For this review, take the finished solid that the model builds, in its own axes (mm). A direction names the side the tool comes from. Round coordinates to 2 decimals unless told otherwise and drop trailing zeros. Write each loop counter-clockwise with the first axis right and the second up, starting at its lowest first coordinate (ties: lowest second). Pieces come first, ordered by that corner, then holes. Notation, with made-up numbers: (-17.5, 67) -> (5.5, 67) arc R13 ccw to (5.5, 83) -> close; hole circle Ø10 at (49.25, 2.25). An arc over 180 degrees is marked (long way). Answer in a Markdown table with one row per item.
Autodesk Inventor part; units mm, degrees
ref_plane "YZ Plane" through (0, 0, 0) normal (1, 0, 0) x (0, 1, 0)
ref_plane "XZ Plane" through (0, 0, 0) normal (0, 1, 0) x (-1, 0, 0)
ref_plane "XY Plane" through (0, 0, 0) normal (0, 0, 1) x (1, 0, 0)
sketch "Sketch1" plane through (0, 0, 0) normal (0, 0, 1) x (1, 0, 0)
  line L0 (0, 0) -> (100, 0)
  line L1 (100, 0) -> (100, 39)
  line L2 (100, 39) -> (0, 39)
  line L3 (0, 39) -> (0, 0)
  dimension "d45" = 100
  dimension "d46" = 39
extrude "bottom" add sketch "Sketch1" along normal blind 3
sketch "Sketch5" plane through (0, 0, 0) normal (0, 0, -1) x (-1, 0, 0)
  line L0 (0, 0) -> (-100, 0)
  line L1 (0, 39) -> (0, 0)
  line L2 (-100, 39) -> (0, 39)
  line L3 (-100, 0) -> (-100, 39)
  line L4 (3, 42) -> (3, -3)
  line L5 (3, -3) -> (-103, -3)
  line L6 (-103, -3) -> (-103, 42)
  line L7 (-103, 42) -> (3, 42)
  dimension "d30" = 3
extrude "walls" add sketch "Sketch5" against normal blind 19.6
sketch "holes" plane through (0, 0, 0) normal (0, 0, 1) x (1, 0, 0)
  line L0 (0, 0) -> (100, 0)
  line L1 (100, 0) -> (100, 39)
  line L2 (100, 39) -> (0, 39)
  line L3 (0, 39) -> (0, 0)
  circle A0 centre (21.5, 34.5) radius 1.55 construction
  circle A1 centre (96.5, 34.5) radius 1.55 construction
  circle A2 centre (96.5, 3.5) radius 1.55 construction
  circle A3 centre (21.5, 3.5) radius 1.55 construction
  line L4 (21.5, 34.5) -> (21.5, 3.5) construction
  line L5 (21.5, 3.5) -> (96.5, 3.5) construction
  line L6 (96.5, 3.5) -> (96.5, 34.5) construction
  line L7 (96.5, 34.5) -> (21.5, 34.5) construction
  dimension "d33" = 3.1
  dimension "d34" = 75
  dimension "d35" = 31
  dimension "d50" = 3.5
  dimension "d51" = 3.5
sketch "Sketch8" plane through (0, 0, 0) normal (0, 0, -1) x (-1, 0, 0)
  line L0 (-95, 6.3) -> (-23, 6.3)
  line L1 (-23, 6.3) -> (-23, 31)
  line L2 (-23, 31) -> (-95, 31)
  line L3 (-95, 31) -> (-95, 6.3)
  line L4 (3, -3) -> (-103, -3)
  line L5 (-96.5, 3.5) -> (-96.5, 34.5) construction
  line L6 (-21.5, 34.5) -> (-21.5, 3.5) construction
  point P0 (0, 0)
  dimension "d99" = 1.5
  dimension "d100" = 1.5
  dimension "d101" = 3.5
  dimension "d102" = 2.8
extrude "display" cut sketch "Sketch8" along normal through all both and the other way through all
sketch "Sketch7" plane through (0, 0, 3) normal (0, 0, 1) x (1, 0, 0)
  circle A0 centre (96.5, 34.5) radius 1.55 construction
  circle A1 centre (21.5, 3.5) radius 1.55 construction
  circle A2 centre (21.5, 34.5) radius 1.55 construction
  arc A3 (23.4365, 31) -> (25.5, 34.5) centre (21.5, 34.5) ccw
  line L0 (15.5, 39) -> (27.5, 39)
  line L1 (0, 39) -> (100, 39)
  arc A4 (27.5, 39) -> (25.5, 37) centre (27.5, 37) ccw
  line L2 (25.5, 37) -> (25.5, 34.5)
  line L3 (16.3235, 0) -> (26.6765, 0)
  line L4 (23, 31) -> (95, 31) construction
  arc A5 (92.6921, 34.5) -> (96.7797, 30.7024) centre (96.5, 34.5) ccw
  line L5 (92.6921, 34.5) -> (92.6921, 36)
  arc A6 (92.6921, 36) -> (89.6921, 39) centre (89.6921, 36) ccw
  line L6 (100, 0) -> (100, 39)
  arc A7 (100, 27.7105) -> (96.7797, 30.7024) centre (97, 27.7105) ccw
  line L7 (100, 39) -> (0, 39)
  line L8 (89.6921, 39) -> (100, 39)
  line L9 (100, 39) -> (100, 27.7105)
  circle A8 centre (96.5, 3.5) radius 3.1765 construction
  line L10 (0, 0) -> (100, 0)
  arc A9 (90.3438, 0) -> (93.3339, 3.2429) centre (90.3438, 3) ccw construction
  arc A10 (96.7571, 6.6661) -> (100, 9.6562) centre (97, 9.6562) ccw construction
  line L11 (100, 9.6562) -> (100, 0)
  line L12 (100, 0) -> (90.3438, 0)
  line L13 (15.5, 39) -> (15.5, 27.8105)
  line L14 (17.0325, 26.964) -> (23.6299, 31.1142)
  line L15 (0, 0) -> (0, 39)
  arc A11 (15.5, 27.8105) -> (17.0325, 26.964) centre (16.5, 27.8105) ccw
  line L16 (100, 0) -> (0, 0)
  line L17 (96.5, 6.6765) -> (95, 6.6765) construction
  line L18 (95, 6.6765) -> (95, 6.3)
  line L19 (23, 6.3) -> (95, 6.3)
  line L20 (95, 6.3) -> (93.3235, 6.3)
  line L21 (93.3235, 6.3) -> (93.3235, 3.5) construction
  line L22 (91.8235, 6.3) -> (91.8235, 2)
  arc A12 (89.8235, 0) -> (91.8235, 2) centre (89.8235, 2) ccw
  line L23 (95, 8.1765) -> (98, 8.1765)
  arc A13 (98, 8.1765) -> (100, 10.1765) centre (98, 10.1765) ccw
  line L24 (100, 39) -> (100, 0)
  line L25 (95, 6.6765) -> (95, 8.1765)
  line L26 (95, 6.3) -> (95, 31) construction
  line L27 (95, 6.3) -> (23, 6.3) construction
  line L28 (26.5, 6.3) -> (26.5, 1.9199)
  arc A14 (26.5, 1.9199) -> (27.9398, 0) centre (28.5, 1.9199) ccw
  line L29 (23, 8.5) -> (18.5, 8.5)
  arc A15 (18.5, 8.5) -> (16.5, 6.5) centre (18.5, 6.5) ccw
  line L30 (16.5, 6.5) -> (16.5, 2)
  arc A16 (14.5, 0) -> (16.5, 2) centre (14.5, 2) ccw
  line L31 (23, 31) -> (23, 6.3)
  line L32 (23, 8.5) -> (23, 6.3)
  line L33 (23, 6.3) -> (26.5, 6.3)
  point P0 (15.5, 26)
  dimension "d54" = 8
  dimension "d61" = 3
  dimension "d62" = 3
  dimension "d65" = 3
  dimension "d66" = 3
  dimension "d81" = 15.5
  dimension "d82" = 13
  dimension "d83" = 1
  dimension "d103" = 1.5
  dimension "d104" = 1.5
  dimension "d105" = 2
  dimension "d106" = 2
  dimension "d117" = 2
  dimension "d118" = 5
  dimension "d119" = 5
  dimension "d120" = 2
  dimension "d121" = 2
  dimension "d122" = 2
  dimension "d123" = 5
extrude "Extrusion19" add sketch "Sketch7" along normal blind 3.8 contours L14 A11 L13 L0 A4 L2 A3 | L31 L19 L28 A14 L10 L3 A16 L30 A15 L29 | L1 L6 A7 A5 L5 A6 | L19 L18 L25 L23 A13 L6 L10 A12 L22
sketch "Sketch9" plane through (0, 0, 0) normal (0, 0, -1) x (-1, 0, 0)
  circle A0 centre (-21.5, 3.5) radius 1.55 construction
  circle A1 centre (-21.5, 34.5) radius 1.55 construction
  circle A2 centre (-21.5, 34.5) radius 3.1
  circle A3 centre (-21.5, 3.5) radius 3.1
  circle A4 centre (-96.5, 34.5) radius 1.55 construction
  circle A5 centre (-96.5, 3.5) radius 1.55 construction
  circle A6 centre (-96.5, 34.5) radius 3.1
  circle A7 centre (-96.5, 3.5) radius 3.1
  line L0 (-95, 6.3) -> (-95, 31)
  point P0 (0, 0)
  point P1 (-94.7478, 6.0573)
  point P2 (-95.3418, 6.3755)
  dimension "d57" = 6.2
  dimension "d58" = 6.2
  dimension "d109" = 6.2
extrude "bolt holes" cut sketch "Sketch9" against normal blind 6.5
sketch "Sketch10" plane through (0, 0, 0) normal (0, 0, -1) x (-1, 0, 0)
  circle A0 centre (-96.5, 34.5) radius 1.55
  circle A1 centre (-96.5, 3.5) radius 1.55
  circle A2 centre (-21.5, 3.5) radius 1.55
  circle A3 centre (-21.5, 34.5) radius 1.55
  point P0 (0, 0)
extrude "holes screws" cut sketch "Sketch10" along normal through all both and the other way through all
sketch "Sketch11" plane through (96.5, 34.5, 6.5) normal (0, 0, -1) x (-1, 0, 0)
  circle A0 centre (75, 0) radius 1.55
  circle A1 centre (75, 0) radius 3.1
  circle A2 centre (75, -31) radius 3.1
  circle A3 centre (0, -31) radius 1.55
  circle A4 centre (0, -31) radius 3.1
  circle A5 centre (0, 0) radius 3.1
  point P0 (96.5, -34.5)
extrude "fill after hole" add sketch "Sketch11" along normal blind 0.6 contours A0 | A1 | A2 | A3 | A4 | A5
sketch "Sketch13" plane through (0, 0, 19.6) normal (0, 0, 1) x (1, 0, 0)
  line L0 (0, 0) -> (0, 39)
  line L1 (0, 39) -> (100, 39)
  line L2 (100, 39) -> (100, 0)
  line L3 (100, 0) -> (0, 0)
  line L4 (-3, 42) -> (-3, -3)
  line L5 (-3, -3) -> (103, -3)
  line L6 (103, -3) -> (103, 42)
  line L7 (103, 42) -> (-3, 42)
  line L8 (-1.7, 40.7) -> (-1.7, -1.7)
  line L9 (-1.7, -1.7) -> (101.7, -1.7)
  line L10 (101.7, -1.7) -> (101.7, 40.7)
  line L11 (101.7, 40.7) -> (-1.7, 40.7)
  dimension "d126" = 1.3
  dimension "d127" = 1.3
  dimension "d128" = 1.3
  dimension "d129" = 1.3
extrude "collar" add sketch "Sketch13" along normal blind 3 contours L7 L6 L5 L4
sketch "Sketch15" plane through (0, 0, 3) normal (0, 0, 1) x (1, 0, 0)
  line L0 (100, 39) -> (0, 39)
  line L1 (0, 39) -> (15.5, 39)
  line L2 (15.5, 39) -> (15.5, 27)
  line L3 (13.5, 25) -> (0, 25)
  line L4 (0, 25) -> (0, 39)
  line L5 (0, 0) -> (0, 39)
  arc A0 (3, 25) -> (0, 22) centre (3, 22) ccw
  line L6 (0, 25) -> (0, 22)
  arc A1 (13.5, 25) -> (15.5, 27) centre (13.5, 27) ccw
  line L7 (14.6154, 25.3399) -> (17.0325, 26.964)
  arc A2 (15.5, 27.8105) -> (17.0325, 26.964) centre (16.5, 27.8105) ccw
  point P0 (15.5, 39)
  point P1 (15.5, 25)
  dimension "d90" = 14
  dimension "d95" = 3
  dimension "d96" = 2
extrude "encoder standoff" add sketch "Sketch15" along normal blind 3
sketch "Sketch12" plane through (0, 0, 0) normal (0, 0, -1) x (-1, 0, 0)
  circle A0 centre (-7.75, 32.5) radius 3.6
  line L0 (0, 0) -> (0, 39)
  line L1 (-7.75, 32.5) -> (-15.5, 32.5) construction
  line L2 (-7.75, 32.5) -> (0, 32.5) construction
  line L3 (0, 39) -> (-100, 39) construction
  line L4 (0, 22) -> (0, 0)
  line L5 (-89.6921, 39) -> (-27.5, 39)
  line L6 (0, 22) -> (0, 39)
  line L7 (0, 39) -> (-15.5, 39)
  line L8 (-15.5, 39) -> (-15.5, 27.8105)
  line L9 (-15.5, 39) -> (-27.5, 39)
  line L10 (-89.6921, 39) -> (-100, 39)
  point P0 (-15.5, 39)
  dimension "d71" = 7.2
  dimension "d112" = 6.5
extrude "encoder hole" cut sketch "Sketch12" along normal through all both and the other way through all
sketch "Sketch14" plane through (0, 0, 0) normal (0, 0, -1) x (-1, 0, 0)
  circle A0 centre (-7.75, 32.5) radius 3.6
  circle A1 centre (-7.75, 32.5) radius 7
  point P0 (0, 0)
  dimension "d87" = 14
extrude "encoder nut" cut sketch "Sketch14" against normal blind 2.5
sketch "Sketch16" plane through (7.75, 32.5, 2.5) normal (0, 0, -1) x (-1, 0, 0)
  circle A0 centre (0, 0) radius 3.6
  point P0 (7.75, -32.5)
extrude "encoder fill before hole" add sketch "Sketch16" against normal blind 0.6
sketch "Sketch18" plane through (0, 0, 6.8) normal (0, 0, 1) x (1, 0, 0)
  circle A0 centre (21.5, 34.5) radius 1.55
  line L0 (15.5, 39) -> (15.5, 27.8105)
  arc A1 (15.5, 27.8105) -> (17.0325, 26.964) centre (16.5, 27.8105) ccw
  line L1 (17.0325, 26.964) -> (23.6299, 31.1142)
  arc A2 (23.6299, 31.1142) -> (25.5, 34.5) centre (21.5, 34.5) ccw
  line L2 (25.5, 34.5) -> (25.5, 37)
  arc A3 (27.5, 39) -> (25.5, 37) centre (27.5, 37) ccw
  line L3 (15.5, 39) -> (27.5, 39)
  circle A4 centre (21.5, 3.5) radius 1.55
  arc A5 (14.5, 0) -> (16.5, 2) centre (14.5, 2) ccw
  line L4 (27.9398, 0) -> (14.5, 0)
  arc A6 (26.5, 1.9199) -> (27.9398, 0) centre (28.5, 1.9199) ccw
  line L5 (26.5, 6.3) -> (26.5, 1.9199)
  line L6 (23, 6.3) -> (26.5, 6.3)
  line L7 (23, 8.5) -> (23, 6.3)
  line L8 (18.5, 8.5) -> (23, 8.5)
  arc A7 (18.5, 8.5) -> (16.5, 6.5) centre (18.5, 6.5) ccw
  line L9 (16.5, 2) -> (16.5, 6.5)
  circle A8 centre (96.5, 3.5) radius 1.55
  line L10 (100, 0) -> (89.8235, 0)
  line L11 (100, 10.1765) -> (100, 0)
  arc A9 (98, 8.1765) -> (100, 10.1765) centre (98, 10.1765) ccw
  line L12 (95, 8.1765) -> (98, 8.1765)
  line L13 (95, 6.3) -> (95, 8.1765)
  line L14 (91.8235, 6.3) -> (95, 6.3)
  line L15 (91.8235, 2) -> (91.8235, 6.3)
  arc A10 (89.8235, 0) -> (91.8235, 2) centre (89.8235, 2) ccw
  circle A11 centre (96.5, 34.5) radius 1.55
  arc A12 (92.6921, 36) -> (89.6921, 39) centre (89.6921, 36) ccw
  line L16 (92.6921, 34.5) -> (92.6921, 36)
  arc A13 (92.6921, 34.5) -> (96.7797, 30.7024) centre (96.5, 34.5) ccw
  arc A14 (100, 27.7105) -> (96.7797, 30.7024) centre (97, 27.7105) ccw
  line L17 (100, 39) -> (100, 27.7105)
  line L18 (89.6921, 39) -> (100, 39)
  point P0 (0, 0)
extrude "Extrusion21" add sketch "Sketch18" along normal blind 0.1
properties part number "top"
1) Consider section B-B on x = 61. State the section outline as (y, z) points.
Solved:
| item | result |
|---|---|
| outline | (-3, 0) -> (6.3, 0) -> (6.3, 3) -> (0, 3) -> (0, 19.6) -> (-1.7, 19.6) -> (-1.7, 22.6) -> (-3, 22.6) -> close; (31, 0) -> (42, 0) -> (42, 22.6) -> (40.7, 22.6) -> (40.7, 19.6) -> (39, 19.6) -> (39, 3) -> (31, 3) -> close |
2) Consider section D-D on x = 7.75. State the section outline as (y, z) points.
Solved:
| item | result |
|---|---|
| outline | (-3, 0) -> (25.5, 0) -> (25.5, 2.5) -> (39.5, 2.5) -> (39.5, 0) -> (42, 0) -> (42, 22.6) -> (40.7, 22.6) -> (40.7, 19.6) -> (39, 19.6) -> (39, 6) -> (36.1, 6) -> (36.1, 3.1) -> (28.9, 3.1) -> (28.9, 6) -> (25, 6) -> (25, 3) -> (0, 3) -> (0, 19.6) -> (-1.7, 19.6) -> (-1.7, 22.6) -> (-3, 22.6) -> close |
3) Consider section C-C on z = 13. State the section outline as (x, y) points, then the cut area to 3 significant figures.
Solved:
| item | result |
|---|---|
| outline | (-3, -3) -> (103, -3) -> (103, 42) -> (-3, 42) -> close; hole (0, 0) -> (100, 0) -> (100, 39) -> (0, 39) -> close |
| area | 870 mm² |
4) Mouldability with a two-part tool opening along X and no side actions: class faces 1 (the flat face through (49, -3, 11)), 2 (the cylindrical face through (15.93, 0.6, 4.92)) as pulls with the +X half, pulls with the -X half, needs draft (parallel to the pull), parting line crosses it, or undercut.
Solved:
| item | result |
|---|---|
| face 1 | needs draft |
| face 2 | undercut |
5) Clearance check with flat-ended pins moving along their axes: pin 1 Ø4 at (x, y) = (21.5, 34.5) entering from -Z; pin 2 Ø1.5 at (x, y) = (21.5, 3) entering from +Z; pin 3 Ø5 at (x, y) = (84, 31.5) entering from +Z. State where each tip first meets the part, or that it passes through.
Solved:
| item | result |
|---|---|
| pin 1 | z = 5.9 |
| pin 2 | z = 6.5 |
| pin 3 | z = 3 |
6) Consider section A-A on y = 17.5. State the section outline as (x, z) points, then the cut area to 3 significant figures.
Solved:
| item | result |
|---|---|
| outline | (-3, 0) -> (23, 0) -> (23, 3) -> (0, 3) -> (0, 19.6) -> (-1.7, 19.6) -> (-1.7, 22.6) -> (-3, 22.6) -> close; (95, 0) -> (103, 0) -> (103, 22.6) -> (101.7, 22.6) -> (101.7, 19.6) -> (100, 19.6) -> (100, 3) -> (95, 3) -> close |
| area | 209 mm² |
7) For line 1 (Y direction, x = 21.5, z = 2.7); line 2 (Y direction, x = 7.75, z = 3.95); line 3 (Y direction, x = 96.5, z = 6.85), list the stretches that pass through material, from the lowest coordinate up. Write a range as [from, to].
Solved:
| item | result |
|---|---|
| line 1 | [-3, 0.4], [6.6, 31.4], [37.6, 42] |
| line 2 | [-3, 0], [25, 28.9], [36.1, 42] |
| line 3 | [-3, 1.95], [5.05, 8.18], [30.69, 32.95], [36.05, 42] |
8) For faces 3 (the flat face through (49, 5, 0)), 4 (the cylindrical face through (21.904, 37.574, 2.909)), 5 (the flat face through (91.824, 4, 5)), list the 3-axis set-ups (+Z, -Z, +X, -X, +Y, -Y) from which the entire face can be reached by the end or side of a thin tool; tool diameter is ignored.
Solved:
| item | result |
|---|---|
| face 3 | -Z, +X, -X, +Y, -Y |
| face 4 | -Z |
| face 5 | +Z |
